from build123d import *

# Parameters (mm, degrees)
F0_W     = 5
F0_H     = 17
F0_W_2   = 3
F0_H_2   = 7.55
F1_DEPTH = 4
F2_DEPTH = 30
F4_DEPTH = 75.711
F5_R     = 1


with BuildPart() as f1:
    # F0 (on Top) → F1 (new body)
    with BuildSketch(Plane.XY):
        with Locations((-35.355, 15.275)):
            Rectangle(F0_W, F0_H)
        Polygon((-34.855, 3.775), (-32.855, 3.775), (-32.855, 6.775), (-37.855, 6.775), (-37.855, 3.775), align=None)
        with Locations((-35.355, -15.275)):
            Rectangle(F0_W, F0_H)
        Polygon((37.855, -3.775), (34.855, -3.775), (32.855, -3.775), (32.855, -6.775), (37.855, -6.775), align=None)
        with Locations((35.355, 15.275)):
            Rectangle(F0_W, F0_H)
        with Locations((-36.355, 0)):
            Rectangle(F0_W_2, F0_H_2)
        Polygon((-32.855, -6.775), (-32.855, -3.775), (-34.855, -3.775), (-37.855, -3.775), (-37.855, -6.775), align=None)
        Polygon((32.855, -3.775), (34.855, -3.775), (34.855, 3.775), (32.855, 3.775), (-32.855, 3.775), (-34.855, 3.775), (-34.855, -3.775), (-32.855, -3.775), align=None)
        with Locations((36.355, 0)):
            Rectangle(F0_W_2, F0_H_2)
        Polygon((32.855, 3.775), (34.855, 3.775), (37.855, 3.775), (37.855, 6.775), (32.855, 6.775), align=None)
        with Locations((35.355, -15.275)):
            Rectangle(F0_W, F0_H)
    extrude(amount=-F1_DEPTH)

    # F0 (on Top) → F2 (join)
    with BuildSketch(Plane.XY):
        Polygon((-34.855, 3.775), (-32.855, 3.775), (-32.855, 6.775), (-37.855, 6.775), (-37.855, 3.775), align=None)
        with Locations((-36.355, 0)):
            Rectangle(F0_W_2, F0_H_2)
        Polygon((-32.855, -6.775), (-32.855, -3.775), (-34.855, -3.775), (-37.855, -3.775), (-37.855, -6.775), align=None)
        Polygon((32.855, 3.775), (34.855, 3.775), (37.855, 3.775), (37.855, 6.775), (32.855, 6.775), align=None)
        with Locations((36.355, 0)):
            Rectangle(F0_W_2, F0_H_2)
        Polygon((37.855, -3.775), (34.855, -3.775), (32.855, -3.775), (32.855, -6.775), (37.855, -6.775), align=None)
    extrude(amount=F2_DEPTH)

    # F3 (on face) → F4 (cut, through all)
    with BuildSketch(Plane.YZ.offset(37.855)):
        Polygon((-23.775, -2), (-6.775, 0), (-23.775, 0), align=None)
        Polygon((23.775, 0), (6.775, 0), (23.775, -2), align=None)
    extrude(amount=-F4_DEPTH, mode=Mode.SUBTRACT)

    # F5
    f5_edges = [f1.edges().sort_by_distance(p)[0] for p in [
        (-37.855, 0, 30),
        (-35.355, -6.775, 30),
        (-37.855, -6.775, 15),
        (35.355, -6.775, 30),
        (37.855, 0, 30),
        (37.855, -6.775, 15),
        (37.855, -15.275, -1),
        (35.355, -23.775, -2),
        (37.855, -23.775, -3),
        (32.855, -23.775, -3),
        (32.855, -15.275, -1),
        (32.855, -6.775, 15),
        (-35.355, -23.775, -2),
        (-37.855, -23.775, -3),
        (-32.855, -23.775, -3),
        (-37.855, -15.275, -1),
        (-32.855, -15.275, -1),
        (-32.855, -6.775, 15),
        (-32.855, -5.275, 30),
        (32.855, -5.275, 30),
        (35.355, 6.775, 30),
        (37.855, 6.775, 15),
        (35.355, -6.775, 0),
        (-35.355, -6.775, 0),
        (35.355, 6.775, 0),
        (37.855, 15.275, -1),
        (35.355, 23.775, -2),
        (32.855, 15.275, -1),
        (37.855, 23.775, -3),
        (32.855, 23.775, -3),
        (-32.855, 15.275, -1),
        (-35.355, 23.775, -2),
        (-37.855, 15.275, -1),
        (-35.355, 6.775, 0),
        (-35.355, 6.775, 30),
        (-32.855, 5.275, 30),
        (-32.855, 23.775, -3),
        (-37.855, 23.775, -3),
        (-32.855, -3.775, -2),
        (32.855, -3.775, -2),
        (-32.855, 3.775, -2),
        (32.855, 3.775, -2),
        (32.855, 5.275, 30),
        (-37.855, 6.775, 15),
        (-32.855, 6.775, 15),
        (32.855, 6.775, 15),
    ]]
    fillet(f5_edges, radius=F5_R)


solid = f1.part
Model file for the job. Use its own axes, mm. A direction names the side the tool comes from. Round coordinates to 2 decimals unless told otherwise and drop trailing zeros. Loops run counter-clockwise (first coordinate to the right, second up) from the corner with the lowest first, then second, coordinate; pieces in that order, holes last. Notation, with made-up numbers: (-31, 82) -> (-12, 82) arc R28 ccw to (-12, 104) -> close; hole circle Ø7 at (40.25, 25). An arc over 180 degrees is marked (long way). Answer as CSV lines item,"result". Start each with the question number.
1) Slice it at C-C (x = -9.5). List the corners of the cut face in (y, z) (3 decimals).
2) Pin check, flat tips, straight feed: P1, Ø4, axis at x = -21, z = 0.5, coming from the -Y side (3 decimals); P2, Ø2.5, axis at x = -36, z = 20, coming from the +Y side (3 decimals); P3, Ø6, axis at y = -6.5, z = 3, coming from the -X side (3 decimals); P4, Ø1, axis at x = 34.5, z = 16.5, coming from the -Y side (3 decimals). Stop position of each tip, or through.
3) Tool access for faces 4 (the face through (35, 6.775, 15)), 5 (the face through (0, 3.775, -2)), 6 (the face through (-32.855, -5.6, 8.8)), 7 (the face through (33.14, 15.133, -1.286)), 8 (the face through (-34.855, 0, 15)): list every direction of +Z, -Z, +X, -X, +Y, -Y with a clear straight run to the whole face (end or side of a thin tool).
4) Slice it at B-B (y = 2). List the corners of the cut face in (x, z) (3 decimals), plus the area to 3 significant figures.
5) Mould opens along X. For faces 1 (the face through (-35, -6.775, 15)), 2 (the face through (34, -3.775, 15)), 3 (the face through (-37.554, 15.348, -1.296)) say: +X half, -X half, draft (parallel to the pull), parting line (faces both ways), or undercut.
6) Probe line 1 along X through (y, z) = (4, 2) (3 decimals); line 2 along Z through (x, y) = (-32, -2); line 3 along X through (y, z) = (6.5, 22.5). List the from-to ranges inside material, lowest first.
7) Slice it at A-A (z = 12). List the corners of the cut face in (x, y) (3 decimals).
Filled in:
1,outline,"(-3.775, -4) -> (3.775, -4) -> (3.775, 0) -> (-3.775, 0) -> close"
2,P1,"stops at y = -3.775"
2,P2,"stops at y = 6.775"
2,P3,"stops at x = -37.855"
2,P4,"stops at y = -6.775"
3,face 4,"+Z, +X, -X, +Y"
3,face 5,"+Z, -Z, +Y"
3,face 6,"+Z, -Y"
3,face 7,"+Z, +Y"
3,face 8,"+Z"
4,outline,"(-37.855, -4) -> (37.855, -4) -> (37.855, 29) arc R1 ccw to (36.855, 30) -> (34.855, 30) -> (34.855, 0) -> (-34.855, 0) -> (-34.855, 30) -> (-36.855, 30) arc R1 ccw to (-37.855, 29) -> close"
4,area,"482 mm2"
5,face 1,"draft"
5,face 2,"undercut"
5,face 3,"-X half"
6,line 1,"x = -37.855 to -32.855, 32.855 to 37.855"
6,line 2,"z = -4 to 0"
6,line 3,"x = -37.54 to -33.17, 33.17 to 37.54"
7,outline,"(-37.855, -5.775) arc R1 ccw to (-36.855, -6.775) -> (-33.855, -6.775) arc R1 ccw to (-32.855, -5.775) -> (-32.855, -3.775) -> (-34.855, -3.775) -> (-34.855, 3.775) -> (-32.855, 3.775) -> (-32.855, 5.775) arc R1 ccw to (-33.855, 6.775) -> (-36.855, 6.775) arc R1 ccw to (-37.855, 5.775) -> close; (32.855, -5.775) arc R1 ccw to (33.855, -6.775) -> (36.855, -6.775) arc R1 ccw to (37.855, -5.775) -> (37.855, 5.775) arc R1 ccw to (36.855, 6.775) -> (33.855, 6.775) arc R1 ccw to (32.855, 5.775) -> (32.855, 3.775) -> (34.855, 3.775) -> (34.855, -3.775) -> (32.855, -3.775) -> close"
